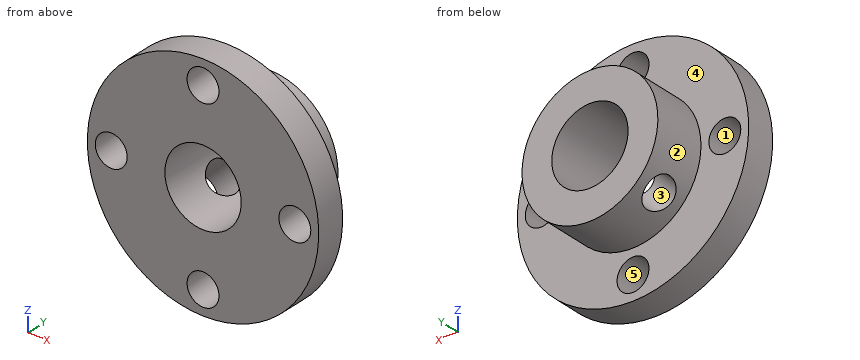
from build123d import *

# Parameters (mm, degrees)
SKETCH1_R                           = 7.239
SKETCH1_R_2                         = 4.064
BOSS_EXTRUDE1_DEPTH                 = 8.89
SKETCH1_3_R                         = 12.319
SKETCH1_3_R_2                       = 7.239
BOSS_EXTRUDE2_DEPTH                 = 3.175
SKETCH2_R                           = 1.7
CUT_EXTRUDE1_DEPTH                  = 3.175
CUT_EXTRUDE2_REACH                  = 27.909
CUT_EXTRUDE2_END_RADIUS             = 4.064
SKETCH5_R                           = 1.7
CUT_EXTRUDE2_DIRECTION_2_REACH      = 27.909
CUT_EXTRUDE2_DIRECTION_2_END_RADIUS = 7.239


with BuildPart() as part:
    # Sketch1 → Boss-Extrude1 (new body)
    with BuildSketch(Plane(origin=(0, 0, 0), x_dir=(1, 0, 0), z_dir=(0, 1, 0))):
        with Locations(Location((0, 0, 0), (0, 0, 270))):
            Circle(SKETCH1_R)
        with Locations(Location((0, 0, 0), (0, 0, 270))):
            Circle(SKETCH1_R_2, mode=Mode.SUBTRACT)
    extrude(amount=BOSS_EXTRUDE1_DEPTH)

    # Sketch1<3> → Boss-Extrude2 (add)
    with BuildSketch(Plane(origin=(0, 0, 0), x_dir=(1, 0, 0), z_dir=(0, 1, 0))):
        with Locations(Location((0, 0, 0), (0, 0, 270))):
            Circle(SKETCH1_3_R)
        with Locations(Location((0, 0, 0), (0, 0, 270))):
            Circle(SKETCH1_3_R_2, mode=Mode.SUBTRACT)
    extrude(amount=BOSS_EXTRUDE2_DEPTH)

    # Sketch2 → Cut-Extrude1 (cut)
    with BuildSketch(Plane(origin=(0, 3.175, 0), x_dir=(1, 0, 0), z_dir=(0, 1, 0))):
        with Locations(Location((0, 9.779, 0), (0, 0, 270))):
            Circle(SKETCH2_R)
        with Locations(Location((9.779, 0, 0), (0, 0, 270))):
            Circle(SKETCH2_R)
        with Locations(Location((0, -9.779, 0), (0, 0, 270))):
            Circle(SKETCH2_R)
        with Locations(Location((-9.779, 0, 0), (0, 0, 270))):
            Circle(SKETCH2_R)
    extrude(amount=-CUT_EXTRUDE1_DEPTH, mode=Mode.SUBTRACT)

    # Cut-Extrude2: up to this cylinder (the profile starts outside it)
    cut_extrude2_end = Plane(origin=(0, 6.0325, 0), z_dir=(0, -1, 0)) * Cylinder(CUT_EXTRUDE2_END_RADIUS, 64.946, mode=Mode.PRIVATE)
    # Sketch5 → Cut-Extrude2 (cut, up to the surface)
    with BuildSketch(Plane(origin=(-4.8895, 0, -4.8895), x_dir=(-0.7071067811865475, 0, 0.7071067811865477), z_dir=(-0.7071067811865477, 0, -0.7071067811865475)), mode=Mode.PRIVATE) as cut_extrude2_sk1:
        with Locations(Location((0, 6.0325, 0), (0, 0, 180))):
            Circle(SKETCH5_R)
    cut_extrude2_tool1 = extrude(cut_extrude2_sk1.sketch, amount=-CUT_EXTRUDE2_REACH, mode=Mode.PRIVATE) - cut_extrude2_end
    add(cut_extrude2_tool1.solids().sort_by_distance((-4.8895, 6.0325, -4.8895))[0], mode=Mode.SUBTRACT)

    # Cut-Extrude2 direction 2: up to this cylinder (the profile starts inside it)
    cut_extrude2_direction_2_end = Plane(origin=(0, 6.0325, 0), z_dir=(0, -1, 0)) * Cylinder(CUT_EXTRUDE2_DIRECTION_2_END_RADIUS, 71.296, mode=Mode.PRIVATE)
    # Sketch5 → Cut-Extrude2 direction 2 (cut, up to the surface)
    with BuildSketch(Plane(origin=(-4.8895, 0, -4.8895), x_dir=(-0.7071067811865475, 0, 0.7071067811865477), z_dir=(-0.7071067811865477, 0, -0.7071067811865475)), mode=Mode.PRIVATE) as cut_extrude2_direction_2_sk1:
        with Locations(Location((0, 6.0325, 0), (0, 0, 180))):
            Circle(SKETCH5_R)
    cut_extrude2_direction_2_tool1 = extrude(cut_extrude2_direction_2_sk1.sketch, amount=CUT_EXTRUDE2_DIRECTION_2_REACH, mode=Mode.PRIVATE) & cut_extrude2_direction_2_end
    add(cut_extrude2_direction_2_tool1.solids().sort_by_distance((-4.8895, 6.0325, -4.8895))[0], mode=Mode.SUBTRACT)


solid = part.part
The model under review builds one solid part; all positions refer to its coordinate system, in mm. Face numbers are marked on the shaded views. A direction names the side the tool comes from. Round coordinates to 2 decimals unless told otherwise and drop trailing zeros. Loops run counter-clockwise (first coordinate to the right, second up) from the corner with the lowest first, then second, coordinate; pieces in that order, holes last. Notation, with made-up numbers: (-37, -38) -> (-24, -38) arc R18 cw to (-24, -19) -> close; hole circle Ø7 at (30, -36.5). An arc over 180 degrees is marked (long way). Return JSON: item names as keys, results as strings.
(1) For the marked faces 1 and 2, list the 3-axis set-ups (+Z, -Z, +X, -X, +Y, -Y) from which the entire face can be reached by the end or side of a thin tool; tool diameter is ignored.
Solved:
{"face 1": "+Y, -Y", "face 2": "+Y"}
(2) Add section B-B on z = 0. Write out the cut boundary in (x, y) (3 decimals).
Solved:
{"outline": "(-12.319, 0) -> (-11.479, 0) -> (-11.479, 3.175) -> (-12.319, 3.175) -> close; (-8.079, 0) -> (-4.064, 0) -> (-4.064, 8.89) -> (-7.239, 8.89) -> (-7.239, 3.175) -> (-8.079, 3.175) -> close; (4.064, 0) -> (8.079, 0) -> (8.079, 3.175) -> (7.239, 3.175) -> (7.239, 8.89) -> (4.064, 8.89) -> close; (11.479, 0) -> (12.319, 0) -> (12.319, 3.175) -> (11.479, 3.175) -> close"}
(3) Add section C-C on z = -10.5. Write out the cut boundary in (x, y) (3 decimals).
Solved:
{"outline": "(-6.443, 0) -> (-1.54, 0) -> (-1.54, 3.175) -> (-6.443, 3.175) -> close; (1.54, 0) -> (6.443, 0) -> (6.443, 3.175) -> (1.54, 3.175) -> close"}
(4) The part is to be moulded in two halves that separate along Y. For the marked faces 3, 4 and 5, say which applies: released by +Y, released by -Y, zero draft, split by the parting line, or undercut.
Solved:
{"face 3": "undercut", "face 4": "released by +Y", "face 5": "zero draft"}
(5) Add section D-D on y = 1.5. Write out the cut boundary in (x, z).
Solved:
{"outline": "circle Ø24.64 at (0, 0); hole circle Ø3.4 at (-9.78, 0); hole circle Ø8.13 at (0, 0); hole circle Ø3.4 at (0, -9.78); hole circle Ø3.4 at (0, 9.78); hole circle Ø3.4 at (9.78, 0)"}
(6) For line 1 (X direction, y = 3, z = 0); line 2 (Z direction, x = -0.75, y = 2.25); line 3 (X direction, y = 6.75, z = 0), list the stretches that pass through material, from the lowest coordinate up.
Solved:
{"line 1": "-12.32 to -11.48, -8.08 to -4.06, 4.06 to 8.08, 11.48 to 12.32", "line 2": "-12.3 to -11.3, -8.25 to -3.99, 3.99 to 8.25, 11.3 to 12.3", "line 3": "-7.24 to -4.06, 4.06 to 7.24"}
(7) For pin 1 (1.5 mm diameter, centred on x = 9, y = 5.5, fed in from +Z); pin 2 (2 mm diameter, centred on y = 4, z = -2.5, fed in from +X); pin 3 (1.5 mm diameter, centred on y = 3.5, z = -1, fed in from +X); pin 4 (4 mm diameter, centred on x = -9, z = -2.5, fed in from +Y) (3 decimals), all flat-tipped, find the tip position at first contact; note any pin that passes through.
Solved:
{"pin 1": "through", "pin 2": "x = 12.17", "pin 3": "x = 12.31", "pin 4": "y = 3.175"}
(8) Add section A-A on x = 0. Write out the cut boundary in (y, z) (3 decimals), plus the area to 3 significant figures.
Solved:
{"outline": "(0, -12.319) -> (3.175, -12.319) -> (3.175, -11.479) -> (0, -11.479) -> close; (0, -8.079) -> (3.175, -8.079) -> (3.175, -7.239) -> (8.89, -7.239) -> (8.89, -4.064) -> (0, -4.064) -> close; (0, 4.064) -> (8.89, 4.064) -> (8.89, 7.239) -> (3.175, 7.239) -> (3.175, 8.079) -> (0, 8.079) -> close; (0, 11.479) -> (3.175, 11.479) -> (3.175, 12.319) -> (0, 12.319) -> close", "area": "67.1 mm2"}
